from build123d import *

# Parameters (mm, degrees)
BOSS_EXTRUDE1_DEPTH = 20
SKETCH2_R           = 2.4
SKETCH2_R_2         = 2.35
BOSS_EXTRUDE2_DEPTH = 3
CUT_EXTRUDE1_DEPTH  = 158.718007744
FILLET1_R           = 3.5


with BuildPart() as part:
    # Sketch1 → Boss-Extrude1 (new body)
    with BuildSketch(Plane(origin=(0, 0, 0), x_dir=(1, 0, 0), z_dir=(0, 1, 0))):
        Polygon((-57.597316241, 51.805869074), (-57.597316241, -8.444130926), (-46.097316241, -28.194130926), (-46.097316241, -108.194130926), (43.902683759, -108.194130926), (43.902683759, -28.194130926), (55.402683759, -8.444130926), (55.402683759, 51.805869074), align=None)
    extrude(amount=BOSS_EXTRUDE1_DEPTH)

    # Sketch2 → Boss-Extrude2 (add)
    with BuildSketch(Plane.XZ):
        with Locations(Location((-51.097316241, -45.305869074, 0), (0, 0, 90))):
            Circle(SKETCH2_R)
        with Locations(Location((48.902683759, -45.305869074, 0), (0, 0, 90))):
            Circle(SKETCH2_R)
        with Locations(Location((-31.847316241, -5.130869074, 0), (0, 0, 90))):
            Circle(SKETCH2_R)
        with Locations(Location((-21.847316241, -5.130869074, 0), (0, 0, 90))):
            Circle(SKETCH2_R)
        with Locations(Location((47.402683759, 6.944130926, 0), (0, 0, 90))):
            Circle(SKETCH2_R_2)
        with Locations(Location((-49.597316241, 6.944130926, 0), (0, 0, 90))):
            Circle(SKETCH2_R_2)
    extrude(amount=BOSS_EXTRUDE2_DEPTH)

    # Sketch3 → Cut-Extrude1 (cut, through all)
    with BuildSketch(Plane(origin=(55.402683759, 0, 0), x_dir=(0, 0, -1), z_dir=(1, 0, 0))):
        Polygon((-108.194130926, 20), (-108.194130926, 2.5), (-8.444130926, 13.563542172), (-8.444130926, 20), align=None)
        Polygon((-8.444130926, 20), (-8.444130926, 13.563542172), (49.587615005, 20), align=None)
        Polygon((49.587615005, 20), (51.805869074, 0), (51.805869074, 20), align=None)
    extrude(amount=-CUT_EXTRUDE1_DEPTH, mode=Mode.SUBTRACT)

    # Fillet1
    fillet1_edges = [part.edges().sort_by_distance(p)[0] for p in [
        (-57.597316241, 10, -50.69674204),
        (55.402683759, 10, -50.69674204),
        (-46.097316241, 5.686508139, 28.194130926),
        (-57.597316241, 6.781771086, 8.444130926),
        (43.902683759, 5.686508139, 28.194130926),
        (43.902683759, 1.25, 108.194130926),
        (-46.097316241, 1.25, 108.194130926),
        (55.402683759, 6.781771086, 8.444130926),
    ]]
    fillet(fillet1_edges, radius=FILLET1_R)


solid = part.part
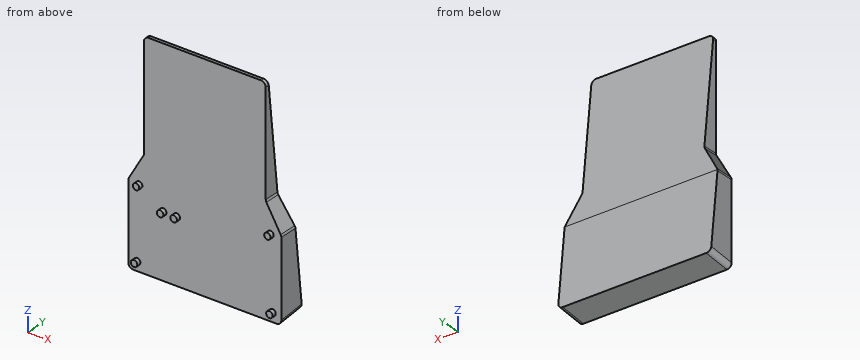
Build history of the part. All positions in model axes, mm. Coordinates: 2 decimals unless noted, no trailing zeros. Write each loop counter-clockwise with the first axis right and the second up, starting at its lowest first coordinate (ties: lowest second). Pieces come first, ordered by that corner, then holes.
(1) Pin check, flat tips, straight feed: pin 1 Ø3 at (x, y) = (-9.5, 15) entering from -Z; pin 2 Ø2 at (x, y) = (33, 2) entering from -Z; pin 3 Ø5.5 at (y, z) = (3, 54.5) entering from -X. Stop position of each tip, or through.
(2) Cut at B-B on z = 78.5. List the corners of the cut face in (x, y).
(3) Drill centre lines: line 1 (X direction, y = 6, z = 51); line 2 (Y direction, x = 40, z = 62.5); line 3 (Y direction, x = 34, z = 32.5). Where is each one in solid material? Low to high.
(4) Cut at C-C on z = 60. List the corners of the cut face in (x, y).
(5) Cut at A-A on x = 38. List the corners of the cut face in (y, z), and give its area (3 significant figures).
Working result:
1. pin 1: stops at z = -50.31
1. pin 2: stops at z = -51.69
1. pin 3: stops at x = -46.1
2. outline: (-46.1, 0) - (43.9, 0) - (43.9, 5.79) - (-46.1, 5.79) - close
3. line 1: x = -46.1 to 43.9
3. line 2: y = 0 to 7.57
3. line 3: y = 0 to 10.9
4. outline: (-46.1, 0) - (43.9, 0) - (43.9, 7.85) - (-46.1, 7.85) - close
5. outline: (0, -51.81) - (20, -49.59) - (2.5, 108.19) - (0, 108.19) - close
5. area: 1,800 mm2
